Input: dimensioned drawing with shaded views. Units: mm. Origin: part minimum x, y, z. A direction names the side the tool comes from. Coordinates: 2 decimals unless noted, no trailing zeros. Loops run counter-clockwise (first coordinate to the right, second up) from the corner with the lowest first, then second, coordinate; pieces in that order, holes last.
Item 1: Section query A-A, the plane y = 15.75. Return the cut outline in (x, z) (1 decimal), then the cut area to 3 significant figures.
Item 2: Pull-direction query (X, two-part tool) for the marked faces 4, 5, 6 and 7; classes: +X half, -X half, draft (parallel to the pull), parting line (faces both ways), or undercut.
Item 3: Section query B-B, the plane z = 12.7. State how many separate pieces and enclosed holes the cut face has, then the cut area to 3 significant figures.
Item 4: Section query D-D, the plane y = 3.5. Return the cut outline in (x, z) (1 decimal).
Item 5: Pin query (flat end, axial travel): pin 1 Ø6.5 at (x, z) = (45.44, 12.7) entering from +Y (3 decimals); pin 2 Ø5 at (y, z) = (9, 9) entering from -X; pin 3 Ø7.5 at (y, z) = (5.56, 12.7) entering from +X; pin 4 Ø4 at (x, z) = (35.5, 6) entering from -Y. Return the tip coordinate at first contact, or that it passes through.
Item 6: Reachability of the marked faces 1, 2 and 3 from +Z, -Z, +X, -X, +Y, -Y: full face, straight path, thin tool, end or side. Return the list, or none.
Item 7: Line query: probe 1 along X at (y, z) = (23.25, 12.7) (1 decimal); probe 2 along X at (y, z) = (9.5, 14.25) (1 decimal); probe 3 along X at (y, z) = (19.75, 14.5) (1 decimal). Output: solid intervals per line, ascending.
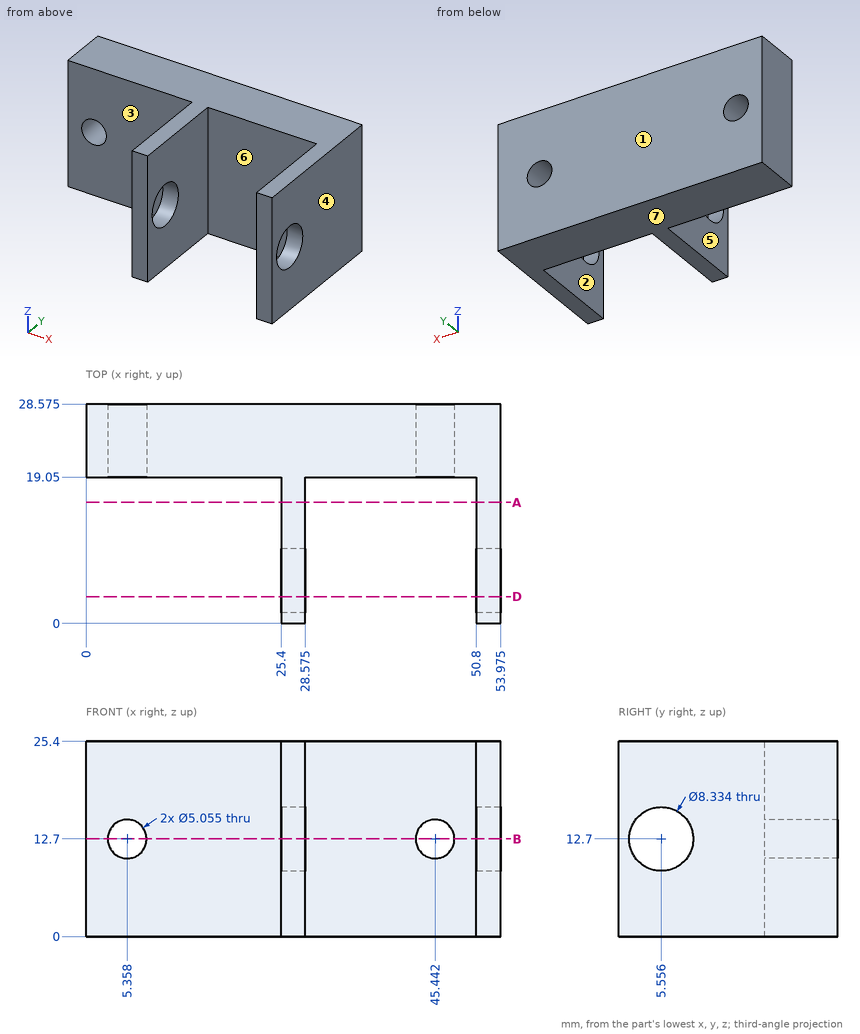
Verdict:
1. outline: (25.4, 0) - (28.6, 0) - (28.6, 25.4) - (25.4, 25.4) - close; (50.8, 0) - (54, 0) - (54, 25.4) - (50.8, 25.4) - close
1. area: 161 mm2
2. face 4: +X half
2. face 5: -X half
2. face 6: undercut
2. face 7: draft
3. separate pieces: 5
3. enclosed holes: 0
3. area: 486 mm2
4. outline: (25.4, 0) - (28.6, 0) - (28.6, 9.1) - (25.4, 9.1) - close; (25.4, 16.3) - (28.6, 16.3) - (28.6, 25.4) - (25.4, 25.4) - close; (50.8, 0) - (54, 0) - (54, 9.1) - (50.8, 9.1) - close; (50.8, 16.3) - (54, 16.3) - (54, 25.4) - (50.8, 25.4) - close
5. pin 1: stops at y = 28.575
5. pin 2: stops at x = 25.4
5. pin 3: passes through
5. pin 4: stops at y = 19.05
6. face 1: +Z, -Z, +X, -X, +Y
6. face 2: +Z, -Z, -Y
6. face 3: +Z, -Z, -X, -Y
7. probe 1: x = 0 to 2.8, 7.9 to 42.9, 48 to 54
7. probe 2: x = 25.4 to 28.6, 50.8 to 54
7. probe 3: x = 0 to 3.6, 7.1 to 43.7, 47.2 to 54
